Design review of the part built by this model. Coordinates are the model's own, in mm. Face numbers are marked on the shaded views. A direction names the side the tool comes from. Coordinates: 2 decimals unless noted, no trailing zeros. Loops run counter-clockwise (first coordinate to the right, second up) from the corner with the lowest first, then second, coordinate; pieces in that order, holes last. Notation, with made-up numbers: (-25.5, 30.5) - (-10.5, 30.5) arc R15 ccw to (-10.5, 44.5) - close; hole circle Ø4 at (79.25, 72.25). An arc over 180 degrees is marked (long way). Use one line per item in the form item = value. Start each with the question number.
(1) Add section D-D (z = -17). State the section outline as (x, y) points.
(2) Add section A-A (x = 0). State the section outline as (y, z) points, plus the area to 3 significant figures.
(3) The part is to be moulded in two halves that separate along X. For the marked faces 1, 2, 3 and 4, say which applies: pulls with the +X half, pulls with the -X half, needs draft (parallel to the pull), parting line crosses it, or undercut.
(4) Add section B-B (y = 18.5). State the section outline as (x, z) points, plus the area to 3 significant figures.
(5) Clearance check with a flat-ended pin moving along its axis: pin 1 Ø6 at (x, z) = (2.5, -40.5) entering from -Y. State where the tip first meets the part, or that it passes through.
(6) For L1, parallel to Y at x = -3, z = -37.5; L2, parallel to X at y = -9, z = -21; L3, parallel to Z at x = 17, y = -15.5, list the stretches that pass through material, from the lowest coordinate up.
(7) Tool access review of the marked faces 5, 6 and 7: name each direction out of +Z, -Z, +X, -X, +Y, -Y from which nothing blocks a thin tool from reaching the whole face with its end or side.
(8) Add section C-C (z = -52.5). State the section outline as (x, y) points.
```python
from build123d import *

# Parameters (mm, degrees)
SKETCH3_W           = 60
SKETCH3_H           = 55
SKETCH3_W_2         = 50
SKETCH3_H_2         = 45
BOSS_EXTRUDE1_DEPTH = 105
SKETCH6_W           = 50
SKETCH6_H           = 5
BOSS_EXTRUDE3_DEPTH = 10
SKETCH7_R           = 2.5
BOSS_EXTRUDE4_DEPTH = 10


with BuildPart() as part:
    # Sketch3 → Boss-Extrude1 (new body)
    with BuildSketch(Plane.XY):
        Rectangle(SKETCH3_W, SKETCH3_H)
        Rectangle(SKETCH3_W_2, SKETCH3_H_2, mode=Mode.SUBTRACT)
    extrude(amount=-BOSS_EXTRUDE1_DEPTH)

    # Sketch6 → Boss-Extrude3 (add)
    with BuildSketch(Plane(origin=(0, -22.5, 0), x_dir=(1, 0, 0), z_dir=(0, 1, 0))):
        with Locations((0, 102.5)):
            Rectangle(SKETCH6_W, SKETCH6_H)
    extrude(amount=BOSS_EXTRUDE3_DEPTH)

    # Sketch7 → Boss-Extrude4 (add)
    with BuildSketch(Plane.XZ.offset(27.5)):
        with Locations((0, -52.5)):
            Circle(SKETCH7_R)
    extrude(amount=BOSS_EXTRUDE4_DEPTH)


solid = part.part
```
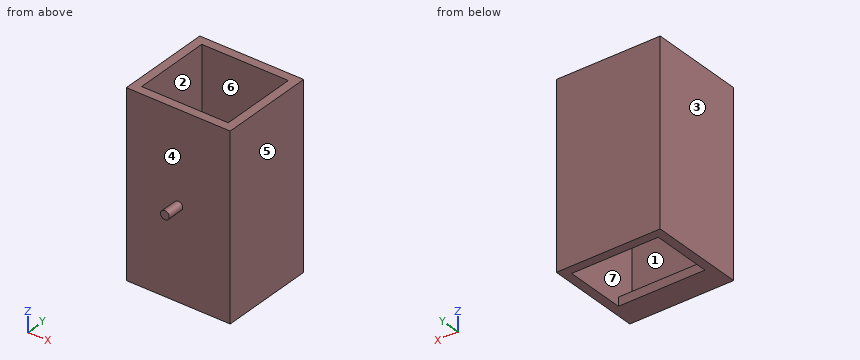
Computed values:
q1.outline = (-30, -27.5) - (30, -27.5) - (30, 27.5) - (-30, 27.5) - close; hole (-25, -22.5) - (25, -22.5) - (25, 22.5) - (-25, 22.5) - close
q2.outline = (-37.5, -55) - (-27.5, -55) - (-27.5, -105) - (-12.5, -105) - (-12.5, -100) - (-22.5, -100) - (-22.5, 0) - (-27.5, 0) - (-27.5, -50) - (-37.5, -50) - close; (22.5, -105) - (27.5, -105) - (27.5, 0) - (22.5, 0) - close
q2.area = 1,150 mm^2
q3.face_1 = undercut
q3.face_2 = undercut
q3.face_3 = pulls with the -X half
q3.face_4 = needs draft
q4.outline = (-30, -105) - (-25, -105) - (-25, 0) - (-30, 0) - close; (25, -105) - (30, -105) - (30, 0) - (25, 0) - close
q4.area = 1,050 mm^2
q5.pin_1 = -27.5
q6.L1 = -27.5 to -22.5, 22.5 to 27.5
q6.L2 = -30 to -25, 25 to 30
q6.L3 = -105 to -100
q7.face_5 = +Z, -Z, +X, +Y, -Y
q7.face_6 = +Z, -Z
q7.face_7 = +Z
q8.outline = (-30, -27.5) - (-2.5, -27.5) - (-2.5, -37.5) - (2.5, -37.5) - (2.5, -27.5) - (30, -27.5) - (30, 27.5) - (-30, 27.5) - close; hole (-25, -22.5) - (25, -22.5) - (25, 22.5) - (-25, 22.5) - close
